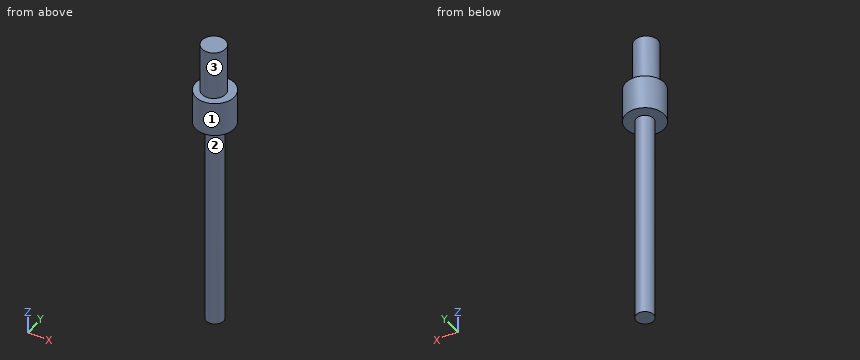
from build123d import *

# Parameters (mm, degrees)
F0_R     = 8.68177
F1_DEPTH = 61.722
F2_R     = 14.1875
F3_DEPTH = 25.4
F4_R     = 6.345818
F5_DEPTH = 156.718


with BuildPart() as f1:
    # F0 (on Top) → F1 (new body)
    with BuildSketch(Plane.XY):
        with Locations((-31.216556, 36.700543)):
            Circle(F0_R)
    extrude(amount=F1_DEPTH)

    # F2 (on Top) → F3 (join)
    with BuildSketch(Plane.XY):
        with Locations((-30.654097, 37.263006)):
            Circle(F2_R)
    extrude(amount=F3_DEPTH)

    # F4 (on face) → F5 (join)
    with BuildSketch(Plane(origin=(0, 0, 0), x_dir=(1, 0, 0), z_dir=(0, 0, -1))):
        with Locations((-30.654097, -37.263006)):
            Circle(F4_R)
    extrude(amount=F5_DEPTH)


solid = f1.part
Geometry check sheet. Reference: the model listing, model coordinates, mm. Face numbers are marked on the shaded views. A direction names the side the tool comes from. Give positions to 0.01 mm unless a question says otherwise; leave off trailing zeros. Loops run counter-clockwise (first coordinate to the right, second up) from the corner with the lowest first, then second, coordinate; pieces in that order, holes last. Notation, with made-up numbers: M 38,-34 L 76,-34 A32 ccw 76,-3 Z; hole C 10,54 d5. An arc over 180 degrees is marked long. Write each question's results on one line, items separated by ' | '.
1) Section check C-C, the plane y = 25.75. Record the boundary of the cut face in (x, z).
Answers follow:
outline: M -38.94,0 L -22.36,0 L -22.36,25.4 L -38.94,25.4 Z
2) Gauge pin test, flat ends, axial feed: pin 1 (12 mm diameter, centred on y = 33.5, z = 6, fed in from -X); pin 2 (5 mm diameter, centred on x = -35, z = -38.5, fed in from -Y); pin 3 (12 mm diameter, centred on y = 29, z = 13, fed in from +X); pin 4 (8 mm diameter, centred on y = 26.5, z = 8.5, fed in from -X). Record the tip position at first contact, or that the pin passes through.
Answers follow:
pin 1: x = -44.84 | pin 2: y = 31.19 | pin 3: x = -16.65 | pin 4: x = -43.13
3) Section check D-D, the plane z = -128. Record the boundary of the cut face in (x, y).
Answers follow:
outline: C -30.65,37.26 d12.69
4) Section check B-B, the plane z = 23. Record the boundary of the cut face in (x, y) (1 decimal).
Answers follow:
outline: C -30.7,37.3 d28.4
5) Tool access check on the marked faces 1, 2 and 3. Record the directions out of +Z, -Z, +X, -X, +Y, -Y that give a thin tool (end or side, any length) a straight path to the whole face; none if there is none.
Answers follow:
face 1: +Z, -Z | face 2: -Z | face 3: +Z
6) Section check A-A, the plane x = -32.25. Record the boundary of the cut face in (y, z), plus the area to 3 significant figures.
Answers follow:
outline: M 23.17,0 L 31.12,0 L 31.12,-156.72 L 43.4,-156.72 L 43.4,0 L 51.36,0 L 51.36,25.4 L 45.32,25.4 L 45.32,61.72 L 28.08,61.72 L 28.08,25.4 L 23.17,25.4 Z | area: 3,270 mm2
7) Thickness scan on line 1 (Z direction, x = -21, y = 43.75); line 2 (X direction, y = 34, z = -100.5); line 3 (Y direction, x = -29, z = -64.5). Record the ranges inside material, lowest first.
Answers follow:
line 1: 0 to 25.4 | line 2: -36.1 to -25.21 | line 3: 31.14 to 43.39
